Print and shaded views of the part. All mm, measured from the part's lowest x, y and z. A direction names the side the tool comes from. Give positions to 0.01 mm unless a question says otherwise; leave off trailing zeros. Write each loop counter-clockwise with the first axis right and the second up, starting at its lowest first coordinate (ties: lowest second). Pieces come first, ordered by that corner, then holes. Notation, with made-up numbers: (52.25, 87.5) -> (109.25, 87.5) arc R22 ccw to (109.25, 112.5) -> close; hole circle Ø2 at (73.25, 22). An arc over 180 degrees is marked (long way). Put each result on its own line as item: value.
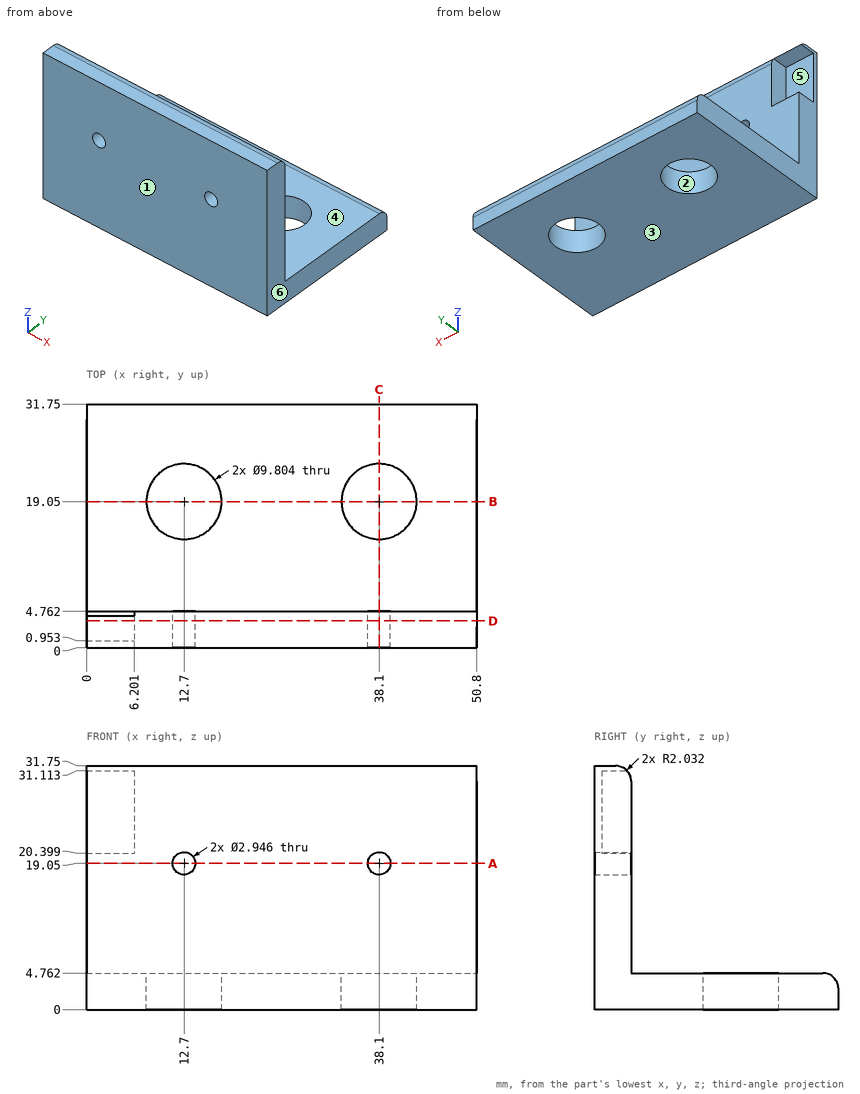
1) Pin check, flat tips, straight feed: pin 1 (7.5 mm diameter, centred on x = 19, y = 23, fed in from +Z); pin 2 (3 mm diameter, centred on x = 4.5, z = 27, fed in from +Y); pin 3 (8 mm diameter, centred on x = 20.5, z = 18.5, fed in from +Y). Stop position of each tip, or through.
Filled sheet:
pin 1: z = 4.76
pin 2: y = 0.95
pin 3: y = 4.76
2) Slice it at C-C (x = 38.1). Give the number of separate pieces and of enclosed holes in the cut face, plus the area to 3 significant figures.
Filled sheet:
separate pieces: 3
enclosed holes: 0
area: 217 mm2
3) Tool access for the marked faces 4, 5 and 6: list every direction of +Z, -Z, +X, -X, +Y, -Y with a clear straight run to the whole face (end or side of a thin tool).
Filled sheet:
face 4: +Z, +X, -X, +Y
face 5: -X, +Y
face 6: +Z, -Z, +X, +Y, -Y
4) Slice it at B-B (y = 19.05). Write the cut outline in (x, z).
Filled sheet:
outline: (0, 0) -> (7.8, 0) -> (7.8, 4.76) -> (0, 4.76) -> close; (17.6, 0) -> (33.2, 0) -> (33.2, 4.76) -> (17.6, 4.76) -> close; (43, 0) -> (50.8, 0) -> (50.8, 4.76) -> (43, 4.76) -> close
5) Wall check: L1, parallel to X at y = 19, z = 1; L2, parallel to X at y = 3.45, z = 19.05; L3, parallel to Y at x = 38, z = 1. Give the ranges that are in metal, low to high.
Filled sheet:
L1: 0 to 7.8, 17.6 to 33.2, 43 to 50.8
L2: 0 to 11.23, 14.17 to 36.63, 39.57 to 50.8
L3: 0 to 14.15, 23.95 to 31.75
6) Pull direction Y, two halves, no side cores. Call the marked faces 1, 2 and 3: released by +Y, released by -Y, zero draft, split by the parting line, or undercut.
Filled sheet:
face 1: released by -Y
face 2: undercut
face 3: zero draft
7) Slice it at A-A (z = 19.05). Write the cut outline in (x, y), plus the area to 3 significant figures.
Filled sheet:
outline: (0, 0) -> (11.23, 0) -> (11.23, 4.76) -> (0, 4.76) -> close; (14.17, 0) -> (36.63, 0) -> (36.63, 4.76) -> (14.17, 4.76) -> close; (39.57, 0) -> (50.8, 0) -> (50.8, 4.76) -> (39.57, 4.76) -> close
area: 214 mm2
8) Slice it at D-D (y = 3.5). Write the cut outline in (x, z).
Filled sheet:
outline: (0, 0) -> (50.8, 0) -> (50.8, 31.6) -> (0, 31.6) -> (0, 31.11) -> (6.2, 31.11) -> (6.2, 20.4) -> (0, 20.4) -> close; hole circle Ø2.95 at (12.7, 19.05); hole circle Ø2.95 at (38.1, 19.05)
